Geometry: final body of the model. Coordinates: model frame, mm. Face numbers are marked on the shaded views. Round coordinates to 2 decimals unless told otherwise and drop trailing zeros. Loops run counter-clockwise (first coordinate to the right, second up) from the corner with the lowest first, then second, coordinate; pieces in that order, holes last. Notation, with made-up numbers: (7.5, 66.5) -> (62.5, 66.5) arc R13 ccw to (62.5, 86.5) -> close; hole circle Ø1 at (3, 74.25). An arc over 180 degrees is marked (long way). Answer in a Markdown table with one row per item.
```python
from build123d import *

# Parameters (mm, degrees)
SKETCH1_W             = 15
SKETCH1_H             = 15
BOSS_EXTRUDE1_DEPTH   = 5
BOSS_EXTRUDE1_2_DEPTH = 5
BOSS_EXTRUDE2_START   = 5
BOSS_EXTRUDE2_DEPTH   = 3
BOSS_EXTRUDE3_START   = -5
BOSS_EXTRUDE3_DEPTH   = 3


with BuildPart() as part:
    # Sketch1 → Boss-Extrude1 (new, symmetric)
    with BuildSketch(Plane.XY):
        with Locations((0, 19.624355653)):
            Rectangle(SKETCH1_W, SKETCH1_H)
    extrude(amount=BOSS_EXTRUDE1_DEPTH, both=True)



with BuildPart() as body_2:
    # Sketch1 → Boss-Extrude1 2 (new, symmetric)
    with BuildSketch(Plane.XY):
        with Locations((0, -19.624355653)):
            Rectangle(SKETCH1_W, SKETCH1_H)
    extrude(amount=BOSS_EXTRUDE1_2_DEPTH, both=True)


with BuildPart() as part_1:
    add(part.part)

    add(body_2.part)  # Boss-Extrude2 merges body 2
    # Sketch1<3> → Boss-Extrude2 (add)
    with BuildSketch(Plane.XY.offset(BOSS_EXTRUDE2_START)):
        Polygon((-6.5, -12.124355653), (0, -0.866025404), (-0.5, 0), (-7.5, -12.124355653), align=None)
        Polygon((0.5, 0), (7.5, 12.124355653), (6.5, 12.124355653), (0, 0.866025404), align=None)
        Polygon((0, -0.866025404), (0.5, 0), (0, 0.866025404), (-0.5, 0), align=None)
    extrude(amount=-BOSS_EXTRUDE2_DEPTH)

    # Sketch1<4> → Boss-Extrude3 (add)
    with BuildSketch(Plane.XY.offset(BOSS_EXTRUDE3_START)):
        Polygon((0, 0.866025404), (-6.5, 12.124355653), (-7.5, 12.124355653), (-0.5, 0), align=None)
        Polygon((7.5, -12.124355653), (0.5, 0), (0, -0.866025404), (6.5, -12.124355653), align=None)
        Polygon((0, -0.866025404), (0.5, 0), (0, 0.866025404), (-0.5, 0), align=None)
    extrude(amount=BOSS_EXTRUDE3_DEPTH)


solid = part_1.part
```
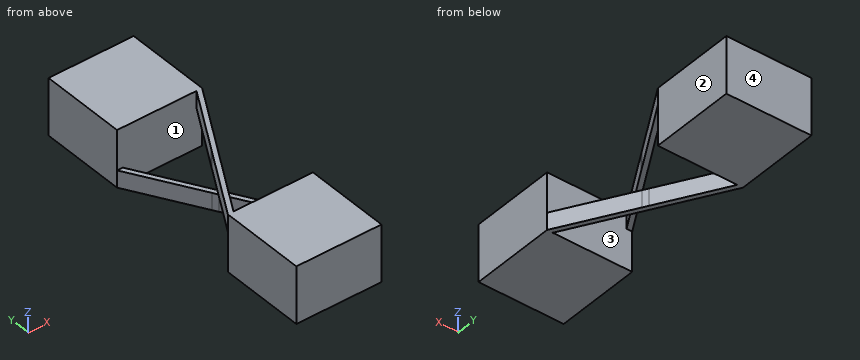
Item 1: Section query D-D, the plane z = -2.5. Output: boundary loops of the cut face in (x, y).
Ans:
| item | result |
|---|---|
| outline | (-7.5, -27.12) -> (7.5, -27.12) -> (7.5, -12.12) -> (-6.5, 12.12) -> (7.5, 12.12) -> (7.5, 27.12) -> (-7.5, 27.12) -> (-7.5, 12.12) -> (6.5, -12.12) -> (-7.5, -12.12) -> close |
Item 2: Mould query, pull axis Y, two halves, no side actions, for the marked faces 1, 2, 3 and 4. Classes: released by +Y, released by -Y, zero draft, split by the parting line, or undercut.
Ans:
| item | result |
|---|---|
| face 1 | undercut |
| face 2 | zero draft |
| face 3 | undercut |
| face 4 | released by +Y |
Item 3: First-contact query: P1, Ø4, axis at y = -8, z = 2.5, coming from the +X side; P2, Ø5, axis at y = 4.5, z = 3, coming from the +X side; P3, Ø7.5, axis at x = -3.5, y = -2, coming from the +Z side. Flat tips, straight axial feed; report the tip coordinate or a pass-through.
Ans:
| item | result |
|---|---|
| P1 | x = -2.96 |
| P2 | x = 4.54 |
| P3 | z = 5 |
Item 4: Section query C-C, the plane y = 1.5. Output: boundary loops of the cut face in (x, z), and give its area (3 significant figures).
Ans:
| item | result |
|---|---|
| outline | (-1.37, -5) -> (-0.37, -5) -> (-0.37, -2) -> (-1.37, -2) -> close; (0.37, 2) -> (1.37, 2) -> (1.37, 5) -> (0.37, 5) -> close |
| area | 6.00 mm2 |
Item 5: Ray query, L1, parallel to Y at x = 2.75, z = 2.5; L2, parallel to Y at x = -5.5, z = 1.5; L3, parallel to Y at x = -3, z = 2.5. Return the intervals inside material, ascending.
Ans:
| item | result |
|---|---|
| L1 | -27.12 to -12.12, 3.9 to 5.63, 12.12 to 27.12 |
| L2 | -27.12 to -12.12, 12.12 to 27.12 |
| L3 | -27.12 to -12.12, -6.06 to -4.33, 12.12 to 27.12 |
Item 6: Section query B-B, the plane x = 2.5. Output: boundary loops of the cut face in (y, z), and give its area (3 significant figures).
Ans:
| item | result |
|---|---|
| outline | (-27.12, -5) -> (-12.12, -5) -> (-12.12, 5) -> (-27.12, 5) -> close; (-5.2, -5) -> (-3.46, -5) -> (-3.46, -2) -> (-5.2, -2) -> close; (3.46, 2) -> (5.2, 2) -> (5.2, 5) -> (3.46, 5) -> close; (12.12, -5) -> (27.12, -5) -> (27.12, 5) -> (12.12, 5) -> close |
| area | 310 mm2 |
Item 7: Section query A-A, the plane z = -0.25. Output: boundary loops of the cut face in (x, y), and give its area (3 significant figures).
Ans:
| item | result |
|---|---|
| outline | (-7.5, -27.12) -> (7.5, -27.12) -> (7.5, -12.12) -> (-7.5, -12.12) -> close; (-7.5, 12.12) -> (7.5, 12.12) -> (7.5, 27.12) -> (-7.5, 27.12) -> close |
| area | 450 mm2 |
